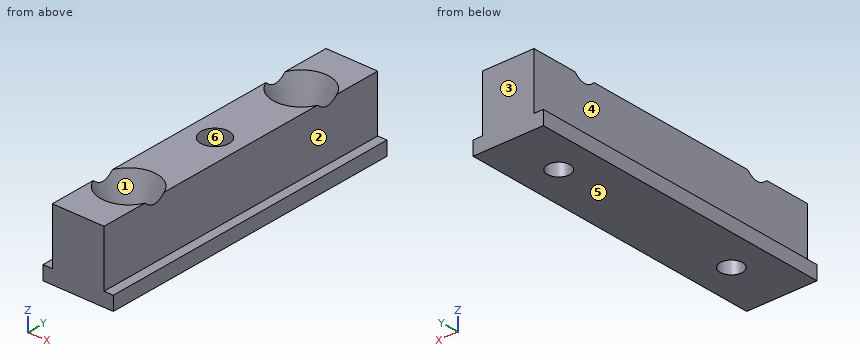
```python
from build123d import *

# Parameters (mm, degrees)
F1_DEPTH       = 11.1
F4_D           = 1.6
F4_CSINK_D     = 4
F4_CSINK_ANGLE = 45
F5_R           = 1
F6_DEPTH       = 3


with BuildPart() as f1:
    # F0 (on Front) → F1 (new body, symmetric)
    with BuildSketch(Plane.XZ):
        Polygon((-2.5, 1), (-2.5, 0), (2.5, 0), (2.5, 1), (1.84, 1), (1.84, 5), (-1.84, 5), (-1.84, 1), align=None)
    extrude(amount=F1_DEPTH, both=True)

    # F4 (through all)
    with Locations(Plane.XY.offset(5)):
        with Locations((0, 7), (0, -7)):
            CounterSinkHole(F4_D / 2, F4_CSINK_D / 2, counter_sink_angle=F4_CSINK_ANGLE)

    # F5 (on face) → F6 (cut)
    with BuildSketch(Plane.XY.offset(5)):
        Circle(F5_R)
    extrude(amount=-F6_DEPTH, mode=Mode.SUBTRACT)


solid = f1.part
```
The model under review builds one solid part; all positions refer to its coordinate system, in mm. Face numbers are marked on the shaded views. A direction names the side the tool comes from. Round coordinates to 2 decimals unless told otherwise and drop trailing zeros. Loops run counter-clockwise (first coordinate to the right, second up) from the corner with the lowest first, then second, coordinate; pieces in that order, holes last. Notation, with made-up numbers: M 59,63 L 118,63 A21 ccw 118,77 Z; hole C 38,59 d9. An arc over 180 degrees is marked long. Write item = value, one per line.
Item 1: For line 1 (Y direction, x = 0, z = 1.25); line 2 (X direction, y = 7, z = 1.4); line 3 (Y direction, x = 0, z = 2.9), list the stretches that pass through material, from the lowest coordinate up. Write a range as [from, to].
Return value:
line_1 = [-11.1, -7.8], [-6.2, 6.2], [7.8, 11.1]
line_2 = [-1.84, -0.8], [0.8, 1.84]
line_3 = [-11.1, -8.13], [-5.87, -1], [1, 5.87], [8.13, 11.1]
Item 2: Take a section at A-A on x = 0. Write out the cut boundary in (y, z), then the cut area to 3 significant figures.
Return value:
outline = M -11.1,0 L -7.8,0 L -7.8,2.1 L -9,5 L -11.1,5 Z; M -6.2,0 L 6.2,0 L 6.2,2.1 L 5,5 L 1,5 L 1,2 L -1,2 L -1,5 L -5,5 L -6.2,2.1 Z; M 7.8,0 L 11.1,0 L 11.1,5 L 9,5 L 7.8,2.1 Z
area = 82.0 mm2
Item 3: Take a section at D-D on z = 2.9. Write out the cut boundary in (x, y), then the cut area to 3 significant figures.
Return value:
outline = M -1.84,-11.1 L 1.84,-11.1 L 1.84,11.1 L -1.84,11.1 Z; hole C 0,-7 d2.26; hole C 0,7 d2.26; hole C 0,0 d2
area = 70.5 mm2
Item 4: Machinability: for the marked faces 4, 5 and 6, which of the approach directions +Z, -Z, +X, -X, +Y, -Y give a long, thin tool a straight path to every point of the face, cutting with its end or side? Answer none if there is none.
Return value:
face_4 = +Z, -X, +Y, -Y
face_5 = -Z, +X, -X, +Y, -Y
face_6 = +Z
Item 5: The part is to be moulded in two halves that separate along X. For the marked faces 1, 2 and 3, say which applies: released by +X, released by -X, zero draft, split by the parting line, or undercut.
Return value:
face_1 = undercut
face_2 = released by +X
face_3 = zero draft
Item 6: Take a section at B-B on z = 1.7. Write out the cut boundary in (x, y), then the cut area to 3 significant figures.
Return value:
outline = M -1.84,-11.1 L 1.84,-11.1 L 1.84,11.1 L -1.84,11.1 Z; hole C 0,-7 d1.6; hole C 0,7 d1.6
area = 77.7 mm2
Item 7: Take a section at C-C on y = 0. Write out the cut boundary in (x, z).
Return value:
outline = M -2.5,0 L 2.5,0 L 2.5,1 L 1.84,1 L 1.84,5 L 1,5 L 1,2 L -1,2 L -1,5 L -1.84,5 L -1.84,1 L -2.5,1 Z
Item 8: Insertion check: P1, Ø1.6, axis at x = 0, y = 0, coming from the +Z side; P2, Ø2, axis at y = -6, z = 3, coming from the -X side; P3, Ø1, axis at y = -5.5, z = 4, coming from the +X side. Each pin has a flat end and moves straight along its axis. Give the tip position at first contact, or say it passes through.
Return value:
P1 = 2
P2 = -1.84
P3 = 1.84
